Design review of the part built by this model. Coordinates are the model's own, in mm. A direction names the side the tool comes from. Coordinates: 2 decimals unless noted, no trailing zeros. Loops run counter-clockwise (first coordinate to the right, second up) from the corner with the lowest first, then second, coordinate; pieces in that order, holes last. Notation, with made-up numbers: M -33.75,-1 L -19.75,-1 A22 cw -19.75,37 Z; hole C 75.5,24.5 d3. An arc over 180 degrees is marked long. Put each result on its own line as item: value. Start each with the question number.
(1) For faces 5 (the flat face through (0, -6.5, -4)), 6 (the flat face through (-4, -6, 16.5)), 7 (the flat face through (0, 6, -4)), list the 3-axis set-ups (+Z, -Z, +X, -X, +Y, -Y) from which the entire face can be reached by the end or side of a thin tool; tool diameter is ignored.
(2) Take a section at A-A, the plane z = -3.75. Give the boundary of the cut face in (x, y), then the cut area to 3 significant figures.
(3) Take a section at C-C, the plane z = 17. Give the boundary of the cut face in (x, y).
(4) The part is to be moulded in two halves that separate along Y. For faces 1 (the cylindrical face through (-6.254, -0.965, -6.999)), 2 (the flat face through (0, -6, -4)), 3 (the flat face through (-6, 0, -4)), 4 (the cylindrical face through (-6.254, 0.965, -6.999)), say which applies: +Y half, -Y half, draft (parallel to the pull), parting line (faces both ways), or undercut.
(5) Clearance check with flat-ended pins moving along their axes: pin 1 (2 mm diameter, centred on y = 0, z = -2.5, fed in from -X); pin 2 (5 mm diameter, centred on y = 6.5, z = 5, fed in from +X); pin 3 (0.6 mm diameter, centred on x = 6.5, z = -1.5, fed in from +Y). State where each tip first meets the part, or that it passes through.
(6) For probe 1 along Z at (x, y) = (-6.75, 3.75); probe 2 along Z at (x, y) = (1.25, 4); probe 3 along Y at (x, z) = (5.5, 9), list the stretches that pass through material, from the lowest coordinate up. Write a range as [from, to].
(7) Take a section at B-B, the plane z = 5. Give the boundary of the cut face in (x, y), then the cut area to 3 significant figures.
```python
from build123d import *

# Parameters (mm, degrees)
SKETCH_1_R      = 7.5
EXTRUDE_1_DEPTH = 14
SKETCH_2_R      = 10
EXTRUDE_2_DEPTH = 2.5
SKETCH_3_R      = 6.8
EXTRUDE_3_DEPTH = 3
SKETCH_4_W      = 0.5
SKETCH_4_H      = 2.5
SKETCH_4_W_2    = 2.5
SKETCH_4_H_2    = 0.5
EXTRUDE_4_DEPTH = 7.3
FILLET_1_R      = 1
FILLET_2_R      = 0.5
FILLET_3_R      = 2


with BuildPart() as part:
    # ｽｹｯﾁ1 → ﾎﾞｽ - 押し出し1 (new body)
    with BuildSketch(Plane.XY):
        Circle(SKETCH_1_R)
    extrude(amount=EXTRUDE_1_DEPTH)

    # ｽｹｯﾁ2 → ﾎﾞｽ - 押し出し2 (add)
    with BuildSketch(Plane.XY.offset(14)):
        Circle(SKETCH_2_R)
    extrude(amount=EXTRUDE_2_DEPTH)

    # ｽｹｯﾁ3 → ﾎﾞｽ - 押し出し3 (add)
    with BuildSketch(Plane.XY.offset(16.5)):
        Circle(SKETCH_3_R)
    extrude(amount=EXTRUDE_3_DEPTH)

    # ｽｹｯﾁ4 → ﾎﾞｽ - 押し出し4 (add)
    with BuildSketch(Plane(origin=(0, 0, 0), x_dir=(-1, 0, 0), z_dir=(0, 0, -1))):
        with Locations((-6.25, 0)):
            Rectangle(SKETCH_4_W, SKETCH_4_H)
        with Locations((6.25, 0)):
            Rectangle(SKETCH_4_W, SKETCH_4_H)
        with Locations((0, 6.25)):
            Rectangle(SKETCH_4_W_2, SKETCH_4_H_2)
        with Locations((0, -6.25)):
            Rectangle(SKETCH_4_W_2, SKETCH_4_H_2)
    extrude(amount=EXTRUDE_4_DEPTH)

    # ﾌｨﾚｯﾄ1
    fillet_1_edges = [part.edges().sort_by_distance(p)[0] for p in [
        (6.25, 1.25, -7.3),
        (6.25, -1.25, -7.3),
        (-6.25, -1.25, -7.3),
        (-6.25, 1.25, -7.3),
        (-1.25, 6.25, -7.3),
        (1.25, 6.25, -7.3),
        (-1.25, -6.25, -7.3),
        (1.25, -6.25, -7.3),
    ]]
    fillet(fillet_1_edges, radius=FILLET_1_R)

    # ﾌｨﾚｯﾄ2
    fillet_2_edges = [part.edges().sort_by_distance(p)[0] for p in [
        (-6.8, 0, 19.5),
    ]]
    fillet(fillet_2_edges, radius=FILLET_2_R)

    # ﾌｨﾚｯﾄ3
    fillet_3_edges = [part.edges().sort_by_distance(p)[0] for p in [
        (-10, 0, 16.5),
    ]]
    fillet(fillet_3_edges, radius=FILLET_3_R)


solid = part.part
```
Computed values:
1. face 5: -Z, +X, -X, -Y
1. face 6: +Z
1. face 7: -Z, +X, -X
2. outline: M -6.5,-1.25 L -6,-1.25 L -6,1.25 L -6.5,1.25 Z; M -1.25,-6.5 L 1.25,-6.5 L 1.25,-6 L -1.25,-6 Z; M -1.25,6 L 1.25,6 L 1.25,6.5 L -1.25,6.5 Z; M 6,-1.25 L 6.5,-1.25 L 6.5,1.25 L 6,1.25 Z
2. area: 5.00 mm^2
3. outline: C 0,0 d13.6
4. face 1: -Y half
4. face 2: undercut
4. face 3: draft
4. face 4: +Y half
5. pin 1: stops at x = -6.5
5. pin 2: stops at x = 6.34
5. pin 3: stops at y = 1.25
6. probe 1: z = [14, 16.5]
6. probe 2: z = [0, 19.5]
6. probe 3: y = [-5.1, 5.1]
7. outline: C 0,0 d15
7. area: 177 mm^2
